Check sheet for the modelled part. Datum: model origin and axes. Units: mm. Face numbers are marked on the shaded views. A direction names the side the tool comes from. Round coordinates to 2 decimals unless told otherwise and drop trailing zeros. Order: outer loops, then holes, each group sorted by start corner. A loop starts at its lowest first (then second) coordinate and runs counter-clockwise, first axis right, second up.
```python
from build123d import *

# Parameters (mm, degrees)
SKETCH_1_R          = 1.29
EXTRUDE_1_DEPTH     = 2.4
SKETCH_5_R          = 2.75
SKETCH_5_R_2        = 1.65
EXTRUDE_4_DEPTH     = 1.6
FILLET_2_R          = 0.36
SKETCH_6_R          = 1.875
CUT_EXTRUDE_1_DEPTH = 0.4
CHAMFER_2_SIZE      = 0.15


with BuildPart() as part:
    # 草图1 → 凸台-拉伸1 (new body)
    with BuildSketch(Plane.XY):
        Polygon((0, 3.175426481), (-2.75, 1.58771324), (-2.75, -1.58771324), (0, -3.175426481), (2.75, -1.58771324), (2.75, 1.58771324), align=None)
        Circle(SKETCH_1_R, mode=Mode.SUBTRACT)
    extrude(amount=-EXTRUDE_1_DEPTH)

    # 草图2 → 切除-旋转1 (revolve, cut)
    with BuildSketch(Plane(origin=(0, 0, 0), x_dir=(0, 0, -1), z_dir=(1, 0, 0))):
        Polygon((0, 2.75), (0.245620093, 3.175426481), (0, 3.175426481), align=None)
        Polygon((2.4, 2.75), (2.154379907, 3.175426481), (2.4, 3.175426481), align=None)
    revolve(axis=Axis((0, 0, 0), (0, 0, -1)), mode=Mode.SUBTRACT)

    # 草图5 → 凸台-拉伸4 (add)
    with BuildSketch(Plane(origin=(0, 0, -2.4), x_dir=(-1, 0, 0), z_dir=(0, 0, -1))):
        Circle(SKETCH_5_R)
        Circle(SKETCH_5_R_2, mode=Mode.SUBTRACT)
    extrude(amount=EXTRUDE_4_DEPTH)

    # 圆角2
    fillet_2_edges = [part.edges().sort_by_distance(p)[0] for p in [
        (2.75, 0, -4),
    ]]
    fillet(fillet_2_edges, radius=FILLET_2_R)

    # 草图6 → 切除-拉伸1 (cut)
    with BuildSketch(Plane(origin=(0, 0, -4), x_dir=(-1, 0, 0), z_dir=(0, 0, -1))):
        Circle(SKETCH_6_R)
    extrude(amount=-CUT_EXTRUDE_1_DEPTH, mode=Mode.SUBTRACT)

    # 倒角2
    chamfer_2_edges = [part.edges().sort_by_distance(p)[0] for p in [
        (-1.29, 0, -2.4),
        (-1.29, 0, 0),
    ]]
    chamfer(chamfer_2_edges, length=CHAMFER_2_SIZE)


solid = part.part
```
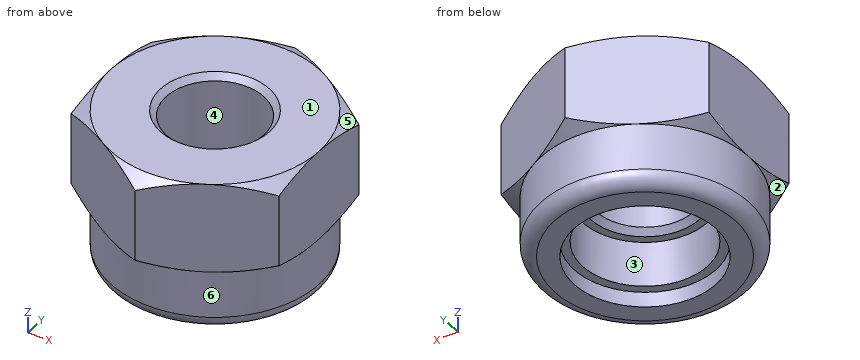
Item 1: Scan lines: line 1 along Y through (x, z) = (0, -3); line 2 along X through (y, z) = (-0.25, -3.45); line 3 along Y through (x, z) = (-1.5, -2.45). Record each from-to range of solid material in increasing order.
Answer:
line 1: y = -2.75 to -1.65, 1.65 to 2.75
line 2: x = -2.74 to -1.63, 1.63 to 2.74
line 3: y = -2.3 to -0.69, 0.69 to 2.3
Item 2: Go/stop test with a flat-tipped pin: P1, Ø3, axis at x = 0, y = 0, coming from the -Z side. Record where the tip stops, or that it passes through.
Answer:
P1: stops at z = -2.4
Item 3: Sectioned sample at B-B (z = -3.15). Record the cut outline in (x, y), and give its area (3 significant figures).
Answer:
outline: circle Ø5.5 at (0, 0); hole circle Ø3.3 at (0, 0)
area: 15.2 mm2
Item 4: Access from +Z, -Z, +X, -X, +Y, -Y to the whole of each face (thin tool, end or side, straight path). Record for the marked faces 5 and 6.
Answer:
face 5: +Z, +X, +Y
face 6: -Z
Item 5: Sectioned sample at A-A (z = -1.55). Record the cut outline in (x, y).
Answer:
outline: (-2.75, -1.59) - (0, -3.18) - (2.75, -1.59) - (2.75, 1.59) - (0, 3.18) - (-2.75, 1.59) - close; hole circle Ø2.58 at (0, 0)
Item 6: Release check for a two-part mould opening along X. For the marked faces 1, 2, 3 and 4 record: released by +X, released by -X, zero draft, split by the parting line, or undercut.
Answer:
face 1: zero draft
face 2: released by -X
face 3: undercut
face 4: undercut
